Input: part model. Units: mm. Frame: model coordinates. A direction names the side the tool comes from. Round coordinates to 2 decimals unless told otherwise and drop trailing zeros. Write each loop counter-clockwise with the first axis right and the second up, starting at its lowest first coordinate (ties: lowest second). Pieces come first, ordered by that corner, then holes. Notation, with made-up numbers: (14.25, 74.25) -> (68.25, 74.25) arc R10 ccw to (68.25, 79.25) -> close; hole circle Ø9 at (-20.5, -26). An arc over 180 degrees is marked (long way). Write item = value, one per line.
```python
from build123d import *

# Parameters (mm, degrees)
SKETCH1_R           = 12.7
BOSS_EXTRUDE1_DEPTH = 38.1
SKETCH2_W           = 5
SKETCH2_H           = 4.000000128
CUT_EXTRUDE2_DEPTH  = 8
SKETCH5_W           = 1
SKETCH5_H           = 20.2
SKETCH5_W_2         = 20.2
SKETCH5_H_2         = 1
BOSS_EXTRUDE2_DEPTH = 38.1


with BuildPart() as part:
    # Sketch1 → Boss-Extrude1 (new body)
    with BuildSketch(Plane(origin=(0, 0, 0), x_dir=(1, 0, 0), z_dir=(0, 1, 0))):
        Circle(SKETCH1_R)
    extrude(amount=BOSS_EXTRUDE1_DEPTH)

    # Sketch2 → Cut-Extrude2 (cut)
    with BuildSketch(Plane(origin=(0, 38.1, 0), x_dir=(1, 0, 0), z_dir=(0, 1, 0))):
        Rectangle(SKETCH2_W, SKETCH2_H)
    extrude(amount=-CUT_EXTRUDE2_DEPTH, mode=Mode.SUBTRACT)

    # Sketch5 → Boss-Extrude2 (add)
    with BuildSketch(Plane(origin=(0, 38.1, 0), x_dir=(1, 0, 0), z_dir=(0, 1, 0))):
        with Locations((0, 12.6)):
            Rectangle(SKETCH5_W, SKETCH5_H)
        with Locations((-12.6, 0)):
            Rectangle(SKETCH5_W_2, SKETCH5_H_2)
        with Locations((12.6, 0)):
            Rectangle(SKETCH5_W_2, SKETCH5_H_2)
        with Locations((0, -12.6)):
            Rectangle(SKETCH5_W, SKETCH5_H)
    extrude(amount=-BOSS_EXTRUDE2_DEPTH)


solid = part.part
```
1) First-contact query: P1, Ø10, axis at y = 33, z = 18, coming from the -X side; P2, Ø4.5, axis at y = 34.5, z = 1, coming from the -X side; P3, Ø1.5, axis at x = -14, y = 25, coming from the -Z side; P4, Ø8, axis at y = 28.5, z = 18.5, coming from the +X side. Flat tips, straight axial feed; report the tip coordinate or a pass-through.
Solutions:
P1 = -0.5
P2 = -22.7
P3 = -0.5
P4 = 0.5
2) Access query for faces 1 (the face through (0, 34, 2)), 2 (the face through (0.5, 19, -18)), 3 (the face through (-0.5, 19, -18)), 4 (the face through (-0.5, 19, 18)). Directions: +Z, -Z, +X, -X, +Y, -Y. A direction counts if a zero-diameter tool reaches every point of the face in a straight line with its end or side. Return the directions, or none.
Solutions:
face_1 = +Y
face_2 = -Z, +X, +Y, -Y
face_3 = -Z, -X, +Y, -Y
face_4 = +Z, -X, +Y, -Y
3) Cut plane D-D (z = -17.5). Return the cut outline in (x, y), and give its area (3 significant figures).
Solutions:
outline = (-0.5, 0) -> (0.5, 0) -> (0.5, 38.1) -> (-0.5, 38.1) -> close
area = 38.1 mm^2
4) Line query: L1, parallel to X at y = 24, z = 14.5; L2, parallel to Z at x = 10, y = 22.5. Output: solid intervals per line, ascending. Write a range as from..to.
Solutions:
L1 = -0.5..0.5
L2 = -7.83..7.83
5) Draft query along X for faces 5 (the face through (0.5, 19, 18)), 6 (the face through (-18, 19, 0.5)), 7 (the face through (0, 30.1, 0)). Return one class per face: +X half, -X half, draft (parallel to the pull), parting line (faces both ways), or undercut.
Solutions:
face_5 = +X half
face_6 = draft
face_7 = undercut
6) Cut plane C-C (y = 5.5). Return the cut outline in (x, z), and give its area (3 significant figures).
Solutions:
outline = (-22.7, -0.5) -> (-12.69, -0.5) arc R12.7 ccw to (-0.5, -12.69) -> (-0.5, -22.7) -> (0.5, -22.7) -> (0.5, -12.69) arc R12.7 ccw to (12.69, -0.5) -> (22.7, -0.5) -> (22.7, 0.5) -> (12.69, 0.5) arc R12.7 ccw to (0.5, 12.69) -> (0.5, 22.7) -> (-0.5, 22.7) -> (-0.5, 12.69) arc R12.7 ccw to (-12.69, 0.5) -> (-22.7, 0.5) -> close
area = 547 mm^2
7) Cut plane B-B (x = -13.5). Return the cut outline in (y, z).
Solutions:
outline = (0, -0.5) -> (38.1, -0.5) -> (38.1, 0.5) -> (0, 0.5) -> close
8) Cut plane A-A (y = 35). Return the cut outline in (x, z), and give its area (3 significant figures).
Solutions:
outline = (-22.7, -0.5) -> (-12.69, -0.5) arc R12.7 ccw to (-0.5, -12.69) -> (-0.5, -22.7) -> (0.5, -22.7) -> (0.5, -12.69) arc R12.7 ccw to (12.69, -0.5) -> (22.7, -0.5) -> (22.7, 0.5) -> (12.69, 0.5) arc R12.7 ccw to (0.5, 12.69) -> (0.5, 22.7) -> (-0.5, 22.7) -> (-0.5, 12.69) arc R12.7 ccw to (-12.69, 0.5) -> (-22.7, 0.5) -> close; hole (-2.5, -2) -> (2.5, -2) -> (2.5, 2) -> (-2.5, 2) -> close
area = 527 mm^2
